For this review, take the finished solid that the model builds, in its own axes (mm). Face numbers are marked on the shaded views. A direction names the side the tool comes from. Coordinates: 2 decimals unless noted, no trailing zeros. Loops run counter-clockwise (first coordinate to the right, second up) from the corner with the lowest first, then second, coordinate; pieces in that order, holes last. Notation, with made-up numbers: (55.25, 23.5) - (98.25, 23.5) arc R17 ccw to (98.25, 43.5) - close; hole circle Ø10 at (38.25, -15). An arc over 180 degrees is marked (long way). Use one line per item in the form item = value. Start each with the question number.
1. Add section A-A on z = 10. Give the boundary of the cut face in (x, y), and give its area (3 significant figures).
2. Machinability: for the marked faces 1 and 2, which of the approach directions +Z, -Z, +X, -X, +Y, -Y give a long, thin tool a straight path to every point of the face, cutting with its end or side? Answer none if there is none.
3. For pin 1 Ø1.5 at (x, y) = (-5.5, 34) entering from +Z; pin 2 Ø24 at (x, y) = (-22.71, 40) entering from +Z; pin 3 Ø18 at (x, z) = (37.29, -15.86) entering from +Y; pin 4 Ø1 at (x, y) = (-28.5, 39.5) entering from +Z, all flat-tipped, find the tip position at first contact; note any pin that passes through.
4. Add section D-D on x = -190.5. Give the boundary of the cut face in (y, z).
5. Add section B-B on x = -77. Give the boundary of the cut face in (y, z).
6. To check wall thickness, follow probe 1 along X at (y, z) = (40, 9); probe 2 along Z at (x, y) = (-22, 51.5); probe 3 along X at (y, z) = (29, -25). State the ranges of each line that lie inside material, in increasing order.
7. Draft analysis for pull direction X (two halves, no side actions). For the marked faces 3, 4, 5 and 6, state which applies: +X half, -X half, draft (parallel to the pull), parting line (faces both ways), or undercut.
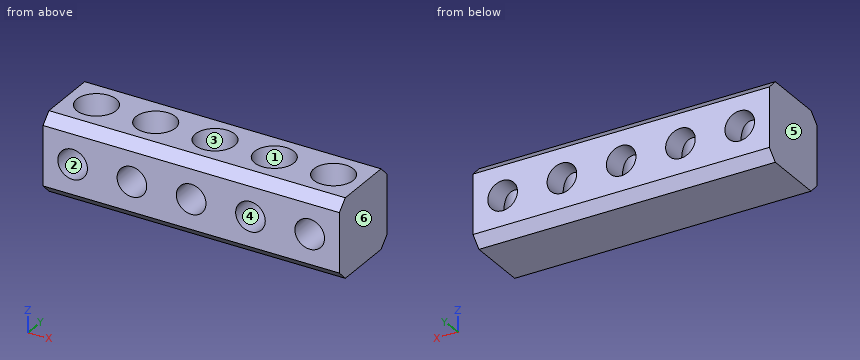
```python
from build123d import *

# Parameters (mm, degrees)
CROQUIS1_W              = 300
CROQUIS1_H              = 80
SALIENTE_EXTRUIR1_DEPTH = 80
CHAFL_N1_SIZE           = 10
CROQUIS2_R              = 20
CORTAR_EXTRUIR1_DEPTH   = 40
CROQUIS3_R              = 15
CORTAR_EXTRUIR2_DEPTH   = 100


with BuildPart() as part:
    # Croquis1 → Saliente-Extruir1 (new body)
    with BuildSketch(Plane(origin=(0, 0, 0), x_dir=(1, 0, 0), z_dir=(0, 1, 0))):
        with Locations((-82.708690096, 15.857316294)):
            Rectangle(CROQUIS1_W, CROQUIS1_H)
    extrude(amount=SALIENTE_EXTRUIR1_DEPTH)

    # Chaflán1
    chafl_n1_edges = [part.edges().sort_by_distance(p)[0] for p in [
        (-82.708690096, 80, 24.142683706),
        (-82.708690096, 0, 24.142683706),
        (-82.708690096, 0, -55.857316294),
        (-82.708690096, 80, -55.857316294),
    ]]
    chamfer(chafl_n1_edges, length=CHAFL_N1_SIZE)

    # Croquis2 → Cortar-Extruir1 (cut)
    with BuildSketch(Plane.XY.offset(24.142683706)):
        with Locations((-82.708690096, 40)):
            Circle(CROQUIS2_R)
        with Locations((-142.708690096, 40)):
            Circle(CROQUIS2_R)
        with Locations((-202.708690096, 40)):
            Circle(CROQUIS2_R)
        with Locations((-22.708690096, 40)):
            Circle(CROQUIS2_R)
        with Locations((37.291309904, 40)):
            Circle(CROQUIS2_R)
    extrude(amount=-CORTAR_EXTRUIR1_DEPTH, mode=Mode.SUBTRACT)

    # Croquis3 → Cortar-Extruir2 (cut, symmetric)
    with BuildSketch(Plane(origin=(0, 80, 0), x_dir=(1, 0, 0), z_dir=(0, 1, 0))):
        with Locations((-82.708690096, 15.857316294)):
            Circle(CROQUIS3_R)
        with Locations((-22.708690096, 15.857316294)):
            Circle(CROQUIS3_R)
        with Locations((37.291309904, 15.857316294)):
            Circle(CROQUIS3_R)
        with Locations((-142.708690096, 15.857316294)):
            Circle(CROQUIS3_R)
        with Locations((-202.708690096, 15.857316294)):
            Circle(CROQUIS3_R)
    extrude(amount=CORTAR_EXTRUIR2_DEPTH, both=True, mode=Mode.SUBTRACT)


solid = part.part
```
Conclusion:
q1.outline = (-232.71, 0) - (67.29, 0) - (67.29, 80) - (-232.71, 80) - close; hole circle Ø40 at (-202.71, 40); hole circle Ø40 at (-142.71, 40); hole circle Ø40 at (-82.71, 40); hole circle Ø40 at (-22.71, 40); hole circle Ø40 at (37.29, 40)
q1.area = 17,700 mm^2
q2.face_1 = +Z
q2.face_2 = +Y, -Y
q3.pin_1 = -15.86
q3.pin_2 = -24.86
q3.pin_3 = through
q3.pin_4 = -29.47
q4.outline = (0, -45.86) - (10, -55.86) - (70, -55.86) - (80, -45.86) - (80, -24.57) - (0, -24.57) - close; (0, -7.14) - (24.16, -7.14) - (24.16, 24.14) - (10, 24.14) - (0, 14.14) - close; (55.84, -7.14) - (80, -7.14) - (80, 14.14) - (70, 24.14) - (55.84, 24.14) - close
q5.outline = (0, -45.86) - (10, -55.86) - (70, -55.86) - (80, -45.86) - (80, -29.73) - (0, -29.73) - close; (0, -1.99) - (20.83, -1.99) - (20.83, 24.14) - (10, 24.14) - (0, 14.14) - close; (59.17, -1.99) - (80, -1.99) - (80, 14.14) - (70, 24.14) - (59.17, 24.14) - close
q6.probe_1 = -232.71 to -222.71, -182.71 to -162.71, -122.71 to -102.71, -62.71 to -42.71, -2.71 to 17.29, 57.29 to 67.29
q6.probe_2 = -55.86 to -30.84
q6.probe_3 = -232.71 to -214.6, -190.82 to -154.6, -130.82 to -94.6, -70.82 to -34.6, -10.82 to 25.4, 49.18 to 67.29
q7.face_3 = undercut
q7.face_4 = undercut
q7.face_5 = -X half
q7.face_6 = +X half
